Geometry check sheet. Reference: the model listing, model coordinates, mm. A direction names the side the tool comes from. Give positions to 0.01 mm unless a question says otherwise; leave off trailing zeros. Loops run counter-clockwise (first coordinate to the right, second up) from the corner with the lowest first, then second, coordinate; pieces in that order, holes last. Notation, with made-up numbers: (1.25, -14.75) -> (31.25, -14.75) arc R17 ccw to (31.25, 13.25) -> close; hole circle Ø7 at (44.25, -34). An arc over 180 degrees is marked (long way). One line per item, written item: value. Start each with the question number.
(1) Sectioned sample at A-A, the plane y = 3.5. Record the cut outline in (x, z) (3 decimals), then the cut area to 3 significant figures.
(2) Scan lines: line 1 along X through (y, z) = (6.25, -46.5); line 2 along X through (y, z) = (5.25, -52); line 3 along Z through (x, y) = (-14.75, 2.25). Record each from-to range of solid material in increasing order. Write a range as from..to.
(3) Sectioned sample at D-D, the plane y = -1. Record the cut outline in (x, z).
(4) Tool access check on faces 1 (the face through (-7.798, -0.838, -52.874)), 2 (the face through (-11, 6, -39.933)), 3 (the face through (-11, 5, -54.433)). Record the directions out of +Z, -Z, +X, -X, +Y, -Y that give a thin tool (end or side, any length) a straight path to the whole face; none if there is none.
(5) Gauge pin test, flat ends, axial feed: pin 1 Ø4 at (x, z) = (-11.5, -44.5) entering from +Y; pin 2 Ø2.5 at (x, z) = (-11, -46.5) entering from +Y; pin 3 Ø4 at (x, z) = (-11.26, -46.43) entering from -Y. Record the tip position at first contact, or that the pin passes through.
(6) Sectioned sample at C-C, the plane z = -46. Record the cut outline in (x, y), then the cut area to 3 significant figures.
(7) Sectioned sample at B-B, the plane x = -7.25. Record the cut outline in (y, z).
(8) Draft check along Z on faces 4 (the face through (-11, 5, -38.433)), 5 (the face through (-7, -1.7, -50)), 6 (the face through (-11, 0, -46)). Enter one of: pulls with the +Z half, pulls with the -Z half, needs draft (parallel to the pull), parting line crosses it, or undercut.
from build123d import *

# Parameters (mm, degrees)
F0_W     = 16
F0_H     = 16
F1_DEPTH = 9.6
F2_R     = 2.5
F3_DEPTH = 1.7
F4_W     = 13
F4_H     = 13
F4_R     = 3.155
F4_R_2   = 2.355
F5_DEPTH = 8


with BuildPart() as f1:
    # F0 (on Front) → F1 (new body)
    with BuildSketch(Plane.XZ):
        with Locations((-11.256055, -46.433249)):
            Rectangle(F0_W, F0_H)
    extrude(amount=-F1_DEPTH)

    # F2 (on face) → F3 (join)
    with BuildSketch(Plane.XZ):
        with Locations((-15.256055, -42.433249)):
            Circle(F2_R)
        with Locations((-15.256055, -50.433249)):
            Circle(F2_R)
        with Locations((-7.256055, -42.433249)):
            Circle(F2_R)
        with Locations((-7.256055, -50.433249)):
            Circle(F2_R)
    extrude(amount=F3_DEPTH)

    # F4 (on face) → F5 (cut)
    with BuildSketch(Plane(origin=(0, 9.6, 0), x_dir=(-1, 0, 0), z_dir=(0, 1, 0))):
        with Locations((11.256055, -46.433249)):
            Rectangle(F4_W, F4_H)
        with Locations((11.256055, -46.433249)):
            Circle(F4_R, mode=Mode.SUBTRACT)
        with Locations((11.256055, -46.433249)):
            Circle(F4_R_2)
    extrude(amount=-F5_DEPTH, mode=Mode.SUBTRACT)


solid = f1.part
Calculated:
1. outline: (-19.256, -54.433) -> (-3.256, -54.433) -> (-3.256, -38.433) -> (-19.256, -38.433) -> close; circle Ø6.31 at (-11.256, -46.433); hole (-17.756, -52.933) -> (-4.756, -52.933) -> (-4.756, -39.933) -> (-17.756, -39.933) -> close; hole circle Ø4.71 at (-11.256, -46.433)
1. area: 101 mm2
2. line 1: x = -19.26..-17.76, -14.41..-13.61, -8.9..-8.1, -4.76..-3.26
2. line 2: x = -19.26..-17.76, -4.76..-3.26
2. line 3: z = -54.43..-52.93, -39.93..-38.43
3. outline: circle Ø5 at (-15.26, -50.43); circle Ø5 at (-15.26, -42.43); circle Ø5 at (-7.26, -50.43); circle Ø5 at (-7.26, -42.43)
4. face 1: -Y
4. face 2: +Y
4. face 3: -Z, +X, -X, +Y, -Y
5. pin 1: stops at y = 9.6
5. pin 2: stops at y = 1.6
5. pin 3: stops at y = 0
6. outline: (-19.26, 0) -> (-3.26, 0) -> (-3.26, 9.6) -> (-4.76, 9.6) -> (-4.76, 1.6) -> (-8.13, 1.6) -> (-8.13, 9.6) -> (-8.94, 9.6) -> (-8.94, 1.6) -> (-13.57, 1.6) -> (-13.57, 9.6) -> (-14.38, 9.6) -> (-14.38, 1.6) -> (-17.76, 1.6) -> (-17.76, 9.6) -> (-19.26, 9.6) -> close
6. area: 62.6 mm2
7. outline: (-1.7, -52.93) -> (0, -52.93) -> (0, -54.43) -> (9.6, -54.43) -> (9.6, -52.93) -> (1.6, -52.93) -> (1.6, -39.93) -> (9.6, -39.93) -> (9.6, -38.43) -> (0, -38.43) -> (0, -39.93) -> (-1.7, -39.93) -> (-1.7, -44.93) -> (0, -44.93) -> (0, -47.93) -> (-1.7, -47.93) -> close
8. face 4: pulls with the +Z half
8. face 5: needs draft
8. face 6: undercut
